```python
from build123d import *

# Parameters (mm, degrees)
PAD004_DEPTH            = 15
SKETCH010_W             = 305
SKETCH010_H             = 30
PAD005_DEPTH            = 60
HOLE002_D               = 5.5
HOLE002_DEPTH           = 57
HOLE002_CBORE_D         = 20
HOLE002_CBORE_DEPTH     = 6.4
PAD006_DEPTH            = 305
SKETCH013_R             = 4.5
HOLE003_DEPTH           = 25
PAD011_DEPTH            = 30
SKETCH026_R             = 2.75
HOLE006_DEPTH           = 230.001
SKETCH027_W             = 30
SKETCH027_H             = 6
POCKET004_DEPTH         = 172
SKETCH028_R             = 10
PAD012_DEPTH            = 30
SKETCH029_R             = 2.75
HOLE007_DEPTH           = 37
BODY005_PLACEMENT_ANGLE = 180


with BuildPart() as part:
    # Sketch009 → Pad004 (new body)
    with BuildSketch(Plane.XY):
        Polygon((-155, 0), (305, 0), (305, 230), (0, 230), (0, 100), (-40, 60), (-155, 60), align=None)
    extrude(amount=PAD004_DEPTH)

    # Sketch010 → Pad005 (join)
    with BuildSketch(Plane.XY):
        with Locations((152.5, 15)):
            Rectangle(SKETCH010_W, SKETCH010_H)
    extrude(amount=PAD005_DEPTH)

    # Hole002
    with Locations(Plane(origin=(0, 30, 0), x_dir=(1, 0, 0), z_dir=(0, 1, 0))):
        with Locations((270, -40), (210, -40), (150, -40), (90, -40), (30, -40)):
            CounterBoreHole(HOLE002_D / 2, HOLE002_CBORE_D / 2, HOLE002_CBORE_DEPTH, depth=HOLE002_DEPTH)

    # Sketch012 → Pad006 (join)
    with BuildSketch(Plane.YZ):
        Polygon((30, 28), (60, 10), (30, 10), align=None)
    extrude(amount=PAD006_DEPTH)

    # Sketch013 → Hole003 (cut)
    with BuildSketch(Plane.XY.offset(15)):
        with Locations((20, 100)):
            Circle(SKETCH013_R)
        with Locations((280, 100)):
            Circle(SKETCH013_R)
        with Locations((150, 100)):
            Circle(SKETCH013_R)
    extrude(amount=-HOLE003_DEPTH, mode=Mode.SUBTRACT)

    # Sketch025 → Pad011 (join)
    with BuildSketch(Plane.XZ.offset(-30)):
        Polygon((-25, 60), (-25, 92), (-57, 92), (-84, 119), (-155, 50), (-155, 0), (10, 0), (10, 60), align=None)
    extrude(amount=-PAD011_DEPTH)

    # Sketch026 → Hole006 (cut, through all)
    with BuildSketch(Plane.XZ):
        with Locations((-50, 85)):
            Circle(SKETCH026_R)
        with Locations((-130, 15)):
            Circle(SKETCH026_R)
    extrude(amount=-HOLE006_DEPTH, mode=Mode.SUBTRACT)

    # Sketch027 → Pocket004 (cut)
    with BuildSketch(Plane.YZ):
        with Locations((15, 13)):
            Rectangle(SKETCH027_W, SKETCH027_H)
    extrude(amount=-POCKET004_DEPTH, mode=Mode.SUBTRACT)

    # Sketch028 → Pad012 (join)
    with BuildSketch(Plane.XY):
        with Locations((63, 218)):
            Circle(SKETCH028_R)
        with Locations((293, 218)):
            Circle(SKETCH028_R)
        with Locations((293, 88)):
            Circle(SKETCH028_R)
        with Locations((63, 88)):
            Circle(SKETCH028_R)
    extrude(amount=PAD012_DEPTH)

    # Sketch029 → Hole007 (cut)
    with BuildSketch(Plane.XY.offset(30)):
        with Locations((63, 218)):
            Circle(SKETCH029_R)
        with Locations((293, 218)):
            Circle(SKETCH029_R)
        with Locations((293, 88)):
            Circle(SKETCH029_R)
        with Locations((63, 88)):
            Circle(SKETCH029_R)
    extrude(amount=-HOLE007_DEPTH, mode=Mode.SUBTRACT)


with BuildPart() as part_1:
    # Body005 placement: moved
    add(part.part.moved(Location((312, -20, -57))).rotate(Axis((312, -20, -57), (0, 0, 1)), BODY005_PLACEMENT_ANGLE))


solid = part_1.part
```
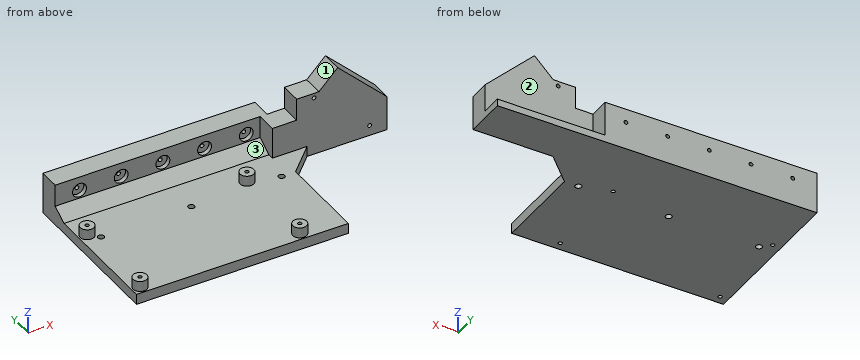
The model under review builds one solid part; all positions refer to its coordinate system, in mm. Face numbers are marked on the shaded views. Round coordinates to 2 decimals unless told otherwise and drop trailing zeros. Loops run counter-clockwise (first coordinate to the right, second up) from the corner with the lowest first, then second, coordinate; pieces in that order, holes last. Notation, with made-up numbers: M 3,-22 L 43,-22 A26 cw 43,10 Z; hole C 48,61.5 d1. An arc over 180 degrees is marked long. Put each result on its own line as item: value.
Q1. For pin 1 (15 mm diameter, centred on x = 381.5, y = -29.5, fed in from +Z); pin 2 (12 mm diameter, centred on x = 289.5, z = -2, fed in from -Y); pin 3 (5.5 mm diameter, centred on x = 162, y = -120, fed in from +Z); pin 4 (16.5 mm diameter, centred on y = -176.5, z = -52, fed in from +X), all flat-tipped, find the tip position at first contact; note any pin that passes through.
Result set:
pin 1: stops at z = -47
pin 2: stops at y = -50
pin 3: passes through
pin 4: stops at x = 312
Q2. Consider section D-D, the plane z = 19. Give the boundary of the cut face in (x, y), then the cut area to 3 significant figures.
Result set:
outline: M 337,-80 L 440.25,-80 L 440.25,-50 L 337,-50 Z
area: 3,100 mm²
Q3. Consider section A-A, the plane y = -64. Give the boundary of the cut face in (x, z), then the cut area to 3 significant figures.
Result set:
outline: M 7,-57 L 467,-57 L 467,-7 L 396,62 L 369,35 L 337,35 L 337,3 L 302,3 L 302,-37.4 L 7,-37.4 Z; hole C 362,28 d5.5; hole C 442,-42 d5.5
area: 19,600 mm²
Q4. Consider section B-B, the plane x = 138. Give the boundary of the cut face in (y, z), then the cut area to 3 significant figures.
Result set:
outline: M -250,-57 L -20,-57 L -20,3 L -50,3 L -50,-29 L -71.67,-42 L -250,-42 Z
area: 4,940 mm²
Q5. Consider section C-C, the plane y = -169. Give the boundary of the cut face in (x, z).
Result set:
outline: M 7,-57 L 312,-57 L 312,-42 L 7,-42 Z
Q6. To check wall thickness, follow L1, parallel to X at y = -47, z = -17; L2, parallel to Y at x = 249, z = -44.5; L3, parallel to X at y = -237.5, z = -31.5. State the ranges of each line that lie inside material, in increasing order.
Result set:
L1: x = 7 to 32, 52 to 92, 112 to 152, 172 to 212, 232 to 272, 292 to 312
L2: y = -250 to -240.75, -235.25 to -110.75, -105.25 to -20
L3: x = 9.01 to 16.3, 21.7 to 28.99, 239.01 to 246.3, 251.7 to 258.99
Q7. Mouldability with a two-part tool opening along Y and no side actions: class the marked faces 1, 2 and 3 as released by +Y, released by -Y, zero draft, split by the parting line, or undercut.
Result set:
face 1: zero draft
face 2: released by +Y
face 3: undercut
